Verification items for the finished model (mm, model axes). Give positions to 0.01 mm unless a question says otherwise; leave off trailing zeros. Order: outer loops, then holes, each group sorted by start corner. A loop starts at its lowest first (then second) coordinate and runs counter-clockwise, first axis right, second up.
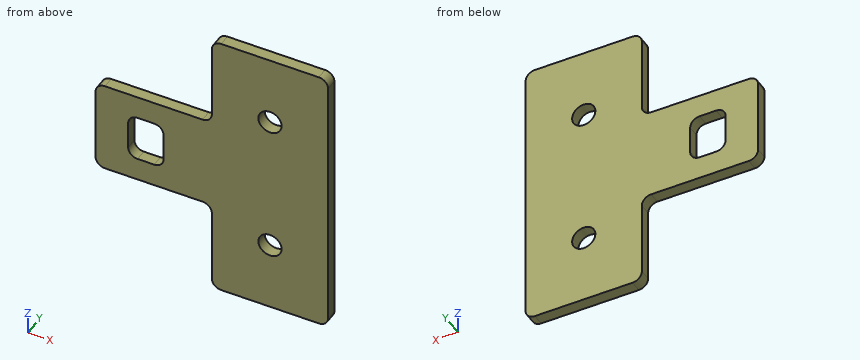
from build123d import *

# Parameters (mm, degrees)
SKETCH1_R           = 3.175
BOSS_EXTRUDE1_DEPTH = 3.175


with BuildPart() as part:
    # Sketch1 → Boss-Extrude1 (new body)
    with BuildSketch(Plane(origin=(0, 0, 0), x_dir=(1, 0, 0), z_dir=(0, 1, 0))):
        with BuildLine():
            Line((2.54, -38.1), (29.21, -38.1))
            ThreePointArc((29.21, -38.1), (31.006051224, -37.356051224), (31.75, -35.56))
            Line((31.75, -35.56), (31.75, 35.56))
            ThreePointArc((31.75, 35.56), (31.006051224, 37.356051224), (29.21, 38.1))
            Line((29.21, 38.1), (2.54, 38.1))
            ThreePointArc((2.54, 38.1), (0.743948776, 37.356051224), (0, 35.56))
            Line((0, 35.56), (0, 15.24))
            ThreePointArc((0, 15.24), (-0.743948776, 13.443948776), (-2.54, 12.7))
            Line((-2.54, 12.7), (-29.21, 12.7))
            ThreePointArc((-29.21, 12.7), (-31.006051224, 11.956051224), (-31.75, 10.16))
            Line((-31.75, 10.16), (-31.75, -10.16))
            ThreePointArc((-31.75, -10.16), (-31.006051224, -11.956051224), (-29.21, -12.7))
            Line((-29.21, -12.7), (-2.54, -12.7))
            ThreePointArc((-2.54, -12.7), (-0.743948776, -13.443948776), (0, -15.24))
            Line((0, -15.24), (0, -35.56))
            ThreePointArc((0, -35.56), (0.743948776, -37.356051224), (2.54, -38.1))
        make_face()
        with Locations(Location((15.875, 19.05, 0), (0, 0, 270))):
            Circle(SKETCH1_R, mode=Mode.SUBTRACT)
        with Locations(Location((15.875, -19.05, 0), (0, 0, 90))):
            Circle(SKETCH1_R, mode=Mode.SUBTRACT)
        with BuildLine():
            Line((-20.32, -6.35), (-15.748, -6.35))
            ThreePointArc((-15.748, -6.35), (-13.951948776, -5.606051224), (-13.208, -3.81))
            Line((-13.208, -3.81), (-13.208, 3.81))
            ThreePointArc((-13.208, 3.81), (-13.951948776, 5.606051224), (-15.748, 6.35))
            Line((-15.748, 6.35), (-20.32, 6.35))
            ThreePointArc((-20.32, 6.35), (-22.116051224, 5.606051224), (-22.86, 3.81))
            Line((-22.86, 3.81), (-22.86, -3.81))
            ThreePointArc((-22.86, -3.81), (-22.116051224, -5.606051224), (-20.32, -6.35))
        make_face(mode=Mode.SUBTRACT)
    extrude(amount=BOSS_EXTRUDE1_DEPTH)


solid = part.part
(1) Section check D-D, the plane z = 33.5. Enter the section's corners in (x, y) (3 decimals), then the cut area to 3 significant figures.
Solved:
outline: (0, 0) - (31.75, 0) - (31.75, 3.175) - (0, 3.175) - close
area: 101 mm2
(2) Section check A-A, the plane y = 0.55. Enter the section's corners in (x, z) (3 decimals).
Solved:
outline: (-31.75, -10.16) arc R2.54 ccw to (-29.21, -12.7) - (-2.54, -12.7) arc R2.54 cw to (0, -15.24) - (0, -35.56) arc R2.54 ccw to (2.54, -38.1) - (29.21, -38.1) arc R2.54 ccw to (31.75, -35.56) - (31.75, 35.56) arc R2.54 ccw to (29.21, 38.1) - (2.54, 38.1) arc R2.54 ccw to (0, 35.56) - (0, 15.24) arc R2.54 cw to (-2.54, 12.7) - (-29.21, 12.7) arc R2.54 ccw to (-31.75, 10.16) - close; hole (-22.86, -3.81) arc R2.54 ccw to (-20.32, -6.35) - (-15.748, -6.35) arc R2.54 ccw to (-13.208, -3.81) - (-13.208, 3.81) arc R2.54 ccw to (-15.748, 6.35) - (-20.32, 6.35) arc R2.54 ccw to (-22.86, 3.81) - close; hole circle Ø6.35 at (15.875, -19.05); hole circle Ø6.35 at (15.875, 19.05)
(3) Section check C-C, the plane x = -5.5. Enter the section's corners in (y, z) (3 decimals).
Solved:
outline: (0, -12.7) - (3.175, -12.7) - (3.175, 12.7) - (0, 12.7) - close
(4) Section check B-B, the plane z = 19.05. Enter the section's corners in (x, y) (3 decimals).
Solved:
outline: (0, 0) - (12.7, 0) - (12.7, 3.175) - (0, 3.175) - close; (19.05, 0) - (31.75, 0) - (31.75, 3.175) - (19.05, 3.175) - close
(5) Scan lines: line 1 (X direction, y = 0.9, z = -19.05); line 2 (Z direction, x = -18, y = 0.7); line 3 (Z direction, x = 17.5, y = 0.9). Record each from-to range of solid material in increasing order.
Solved:
line 1: x = 0 to 12.7, 19.05 to 31.75
line 2: z = -12.7 to -6.35, 6.35 to 12.7
line 3: z = -38.1 to -21.78, -16.32 to 16.32, 21.78 to 38.1
(6) Go/stop test with flat-tipped pins: pin 1 (1 mm diameter, centred on y = 1.5, z = 29.5, fed in from -X); pin 2 (5 mm diameter, centred on x = 15.875, z = -19.05, fed in from +Y); pin 3 (1 mm diameter, centred on x = -15.5, y = 1.5, fed in from +Z); pin 4 (10 mm diameter, centred on x = -16, z = 14.5, fed in from +Y) (3 decimals). Record where each tip stops, or that it passes through.
Solved:
pin 1: stops at x = 0
pin 2: passes through
pin 3: stops at z = 12.7
pin 4: stops at y = 3.175
